Autodesk Inventor part; units mm, degrees
ref_plane "YZ Plane" through (0, 0, 0) normal (1, 0, 0) x (0, 1, 0)
ref_plane "XZ Plane" through (0, 0, 0) normal (0, 1, 0) x (-1, 0, 0)
ref_plane "XY Plane" through (0, 0, 0) normal (0, 0, 1) x (1, 0, 0)
sketch "スケッチ1" plane through (0, 0, 0) normal (0, 0, 1) x (1, 0, 0)
  circle A0 centre (0, 0) radius 17
  dimension "d0" = 34
extrude "押し出し1" add sketch "スケッチ1" along normal blind 73
sketch "スケッチ2" plane through (0, 0, 73) normal (0, 0, 1) x (1, 0, 0)
  line L0 (-21.5, 21.5) -> (21.5, 21.5)
  line L1 (21.5, 21.5) -> (21.5, -21.5)
  line L2 (21.5, -21.5) -> (-21.5, -21.5)
  line L3 (-21.5, -21.5) -> (-21.5, 21.5)
  line L4 (-21.5, 21.5) -> (21.5, -21.5) construction
  line L5 (21.5, 21.5) -> (-21.5, -21.5) construction
  point P0 (0, 0)
  dimension "d3" = 43
  dimension "d4" = 43
extrude "押し出し2" add sketch "スケッチ2" along normal blind 18.5
sketch "スケッチ3" plane through (0, 0, 91.5) normal (0, 0, 1) x (1, 0, 0)
  circle A0 centre (0, 0) radius 40
  dimension "d7" = 80
extrude "押し出し3" add sketch "スケッチ3" along normal blind 9
sketch "スケッチ4" plane through (0, 0, 100.5) normal (0, 0, 1) x (1, 0, 0)
  circle A0 centre (0, 0) radius 30.5
  dimension "d10" = 61
extrude "押し出し4" add sketch "スケッチ4" along normal blind 4.5
sketch "スケッチ5" plane through (0, 0, 105) normal (0, 0, 1) x (1, 0, 0)
  circle A0 centre (0, 0) radius 27.5
  dimension "d13" = 55
extrude "押し出し5" add sketch "スケッチ5" along normal blind 15
sketch "スケッチ6" plane through (0, 0, 120) normal (0, 0, 1) x (1, 0, 0)
  circle A0 centre (0, 0) radius 6
  dimension "d16" = 12
extrude "押し出し6" add sketch "スケッチ6" along normal blind 21
sketch "スケッチ7" plane through (0, 0, 100.5) normal (0, 0, 1) x (1, 0, 0)
  circle A0 centre (0, 0) radius 34.5 construction
  circle A1 centre (-34.5, 0) radius 2
  circle A2 centre (0, -34.5) radius 2
  circle A3 centre (34.5, 0) radius 2
  circle A4 centre (0, 34.5) radius 2
  dimension "d19" = 69
  dimension "d20" = 4
  dimension "d23" = 360
extrude "押し出し7" cut sketch "スケッチ7" against normal blind 9
sketch "スケッチ8" plane through (0, 0, 100.5) normal (0, 0, 1) x (1, 0, 0)
  circle A0 centre (0, 0) radius 34.5 construction
  circle A1 centre (-34.5, 0) radius 4
  circle A2 centre (0, -34.5) radius 4
  circle A3 centre (34.5, 0) radius 4
  circle A4 centre (0, 34.5) radius 4
  dimension "d27" = 69
  dimension "d28" = 8
  dimension "d31" = 360
extrude "押し出し8" cut sketch "スケッチ8" against normal blind 4
properties part number "TukasaMoter"
For this review, take the finished solid that the model builds, in its own axes (mm). A direction names the side the tool comes from. Round coordinates to 2 decimals unless told otherwise and drop trailing zeros. Order: outer loops, then holes, each group sorted by start corner. A loop starts at its lowest first (then second) coordinate and runs counter-clockwise, first axis right, second up. Notation, with made-up numbers: (0.5, -32) -> (42.5, -32) arc R22 cw to (42.5, -7) -> close; hole circle Ø10 at (72.25, -7). An arc over 180 degrees is marked (long way). Use a Markdown table: item, result.
Item 1: Take a section at D-D (y = -7.5). State the section outline as (x, z) points, plus the area to 3 significant figures.
Resolved:
| item | result |
|---|---|
| outline | (-39.29, 91.5) -> (-21.5, 91.5) -> (-21.5, 73) -> (-15.26, 73) -> (-15.26, 0) -> (15.26, 0) -> (15.26, 73) -> (21.5, 73) -> (21.5, 91.5) -> (39.29, 91.5) -> (39.29, 100.5) -> (29.56, 100.5) -> (29.56, 105) -> (26.46, 105) -> (26.46, 120) -> (-26.46, 120) -> (-26.46, 105) -> (-29.56, 105) -> (-29.56, 100.5) -> (-39.29, 100.5) -> close |
| area | 4,790 mm² |
Item 2: For line 1 along Y through (x, z) = (0, 93.95); line 2 along Y through (x, z) = (0, 97.55); line 3 along Z through (x, y) = (-23.5, -20.5), list the stretches that pass through material, from the lowest coordinate up. Write a range as [from, to].
Resolved:
| item | result |
|---|---|
| line 1 | y = [-40, -36.5], [-32.5, 32.5], [36.5, 40] |
| line 2 | y = [-40, -38.5], [-30.5, 30.5], [38.5, 40] |
| line 3 | z = [91.5, 100.5] |
Item 3: Machinability: for faces 1 (the flat face through (-4.7, 27.3, 105)), 2 (the cylindrical face through (9.139, -14.334, 35.989)), 3 (the flat face through (0, 21.5, 82)), 4 (the flat face through (21.5, 0, 82)), which of the approach directions +Z, -Z, +X, -X, +Y, -Y give a long, thin tool a straight path to every point of the face, cutting with its end or side? Answer none if there is none.
Resolved:
| item | result |
|---|---|
| face 1 | +Z |
| face 2 | -Z |
| face 3 | -Z, +X, -X, +Y |
| face 4 | -Z, +X, +Y, -Y |
Item 4: Take a section at A-A (y = 34.5). State the section outline as (x, z) points.
Resolved:
| item | result |
|---|---|
| outline | (-20.24, 91.5) -> (-2, 91.5) -> (-2, 96.5) -> (-4, 96.5) -> (-4, 100.5) -> (-20.24, 100.5) -> close; (2, 91.5) -> (20.24, 91.5) -> (20.24, 100.5) -> (4, 100.5) -> (4, 96.5) -> (2, 96.5) -> close |
Item 5: For pin 1 (5 mm diameter, centred on x = 34.5, y = 0, fed in from +Z); pin 2 (1 mm diameter, centred on x = -8.5, z = 56.5, fed in from +Y); pin 3 (1.5 mm diameter, centred on x = 4.5, z = 82.5, fed in from +Y), all flat-tipped, find the tip position at first contact; note any pin that passes through.
Resolved:
| item | result |
|---|---|
| pin 1 | stops at z = 96.5 |
| pin 2 | stops at y = 15 |
| pin 3 | stops at y = 21.5 |
Item 6: Draft analysis for pull direction Y (two halves, no side actions). For faces 5 (the flat face through (0, -21.5, 82)), 6 (the cylindrical face through (-8.67, 39.05, 95.94)), 7 (the cylindrical face through (-0.434, 32.548, 94.035)), state which applies: +Y half, -Y half, draft (parallel to the pull), parting line (faces both ways), or undercut.
Resolved:
| item | result |
|---|---|
| face 5 | -Y half |
| face 6 | parting line |
| face 7 | undercut |
Item 7: Take a section at C-C (z = 64.5). State the section outline as (x, y) points.
Resolved:
| item | result |
|---|---|
| outline | circle Ø34 at (0, 0) |
